Source: CAD feature listing. Evaluate the final solid. Frame: model axes, mm. Face numbers are marked on the shaded views. Give positions to 0.01 mm unless a question says otherwise; leave off trailing zeros. Order: outer loops, then holes, each group sorted by start corner. A loop starts at its lowest first (then second) coordinate and runs counter-clockwise, first axis right, second up.
1) Section C-C, the plane z = 1.25. Return loops of the section in (x, y) (3 decimals).
2) Section D-D, the plane z = 2. Return loops of the section in (x, y) (3 decimals), plus the area to 3 significant figures.
3) Material intervals for line 1 (Y direction, x = 0, z = 3.25) (3 decimals); line 2 (X direction, y = 0, z = 3); line 3 (X direction, y = 2.5, z = 2), sorted ascending.
4) Section B-B, the plane y = 1.5. Return loops of the section in (x, z).
5) Section A-A, the plane x = 2.5. Return loops of the section in (y, z).
6) Draft query along X for the marked faces 1, 2 and 3. Return one class per face: released by +X, released by -X, zero draft, split by the parting line, or undercut.
7) First-contact query: P1, Ø2, axis at y = -3.5, z = 1, coming from the -X side; P2, Ø1.5, axis at x = 3, y = -3.5, coming from the +Z side; P3, Ø4, axis at x = -0.5, z = 4, coming from the +Y side (3 decimals); P4, Ø3, axis at x = -0.5, y = 2, coming from the +Z side. Flat tips, straight axial feed; report the tip coordinate or a pass-through.
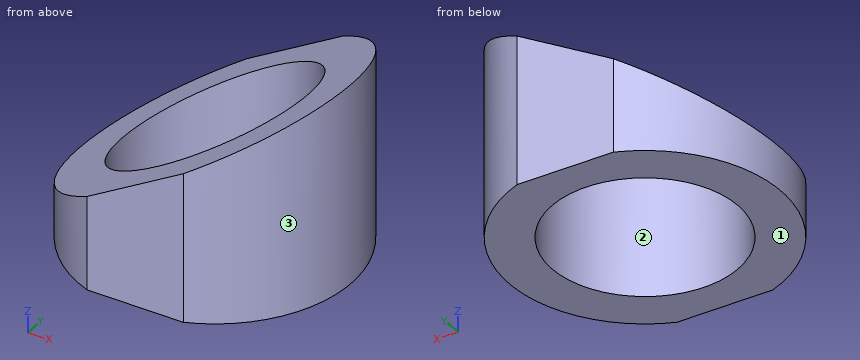
```python
from build123d import *

# Parameters (mm, degrees)
F0_R          = 4.75
F0_R_2        = 3.25
F1_DEPTH      = 10
F3_DEPTH      = 4.751
F3_DEPTH_BACK = 4.751
F5_DEPTH      = 6.9858275573


with BuildPart() as f1:
    # F0 (on Top) → F1 (new body)
    with BuildSketch(Plane.XY):
        Circle(F0_R)
        Circle(F0_R_2, mode=Mode.SUBTRACT)
    extrude(amount=F1_DEPTH)

    # F2 (on Front) → F3 (cut, two sides)
    with BuildSketch(Plane.XZ) as f3_sk:
        Polygon((4.75, 10), (-4.75, 10), (-4.75, 1.5), (4.75, 6.9848275573), align=None)
    extrude(amount=-F3_DEPTH, mode=Mode.SUBTRACT)
    extrude(f3_sk.sketch, amount=F3_DEPTH_BACK, mode=Mode.SUBTRACT)

    # F4 (on face) → F5 (cut, through all)
    with BuildSketch(Plane(origin=(0, 0, 0), x_dir=(1, 0, 0), z_dir=(0, 0, -1))):
        with BuildLine():
            Line((-1.6746566812, 4.445), (1.6746566812, 4.445))
            ThreePointArc((1.6746566812, 4.445), (0, 4.75), (-1.6746566812, 4.445))
        make_face()
        with BuildLine():
            Line((1.6746566812, -4.445), (-1.6746566812, -4.445))
            ThreePointArc((-1.6746566812, -4.445), (0, -4.75), (1.6746566812, -4.445))
        make_face()
    extrude(amount=-F5_DEPTH, mode=Mode.SUBTRACT)


solid = f1.part
```
From the geometry:
1. outline: (-1.675, -4.445) - (1.675, -4.445) arc R4.75 ccw to (1.675, 4.445) - (-1.675, 4.445) arc R4.75 ccw to start; hole circle Ø6.5 at (0, 0)
2. outline: (-3.884, -2.734) arc R4.75 ccw to (-1.675, -4.445) - (1.675, -4.445) arc R4.75 ccw to (1.675, 4.445) - (-1.675, 4.445) arc R4.75 ccw to (-3.884, 2.734) - close; hole circle Ø6.5 at (0, 0)
2. area: 33.1 mm2
3. line 1: y = -4.445 to -3.25, 3.25 to 4.445
3. line 2: x = 3.25 to 4.75
3. line 3: x = -3.88 to -2.08, 2.08 to 4.04
4. outline: (-4.51, 0) - (-2.88, 0) - (-2.88, 2.58) - (-4.51, 1.64) - close; (2.88, 0) - (4.51, 0) - (4.51, 6.84) - (2.88, 5.91) - close
5. outline: (-4.04, 0) - (-2.08, 0) - (-2.08, 5.69) - (-4.04, 5.69) - close; (2.08, 0) - (4.04, 0) - (4.04, 5.69) - (2.08, 5.69) - close
6. face 1: zero draft
6. face 2: undercut
6. face 3: released by +X
7. P1: stops at x = -4.04
7. P2: stops at z = 6.33
7. P3: stops at y = 4.445
7. P4: stops at z = 4.45
